Can you work these out from the model? Positions are in its coordinate system, mm. A direction names the side the tool comes from. Round coordinates to 2 decimals unless told otherwise and drop trailing zeros. Loops run counter-clockwise (first coordinate to the right, second up) from the corner with the lowest first, then second, coordinate; pieces in that order, holes last. Notation, with made-up numbers: M 80.5,70 L 122.5,70 A21 ccw 122.5,85 Z; hole C 56.25,70.5 d2. An arc over 180 degrees is marked long. Use a Markdown table: item, result. Add a question column.
```python
from build123d import *

# Parameters (mm, degrees)
F1_DEPTH = 12.7
F2_SCALE = 0.66


with BuildPart() as f1:
    # F0 (on Top) → F1 (new body)
    with BuildSketch(Plane.XY):
        with BuildLine():
            ThreePointArc((9.144, -75.649370546), (57.0228585744, -50.545361805), (76.2, 0))
            ThreePointArc((76.2, 0), (-50.545361805, 57.0228585744), (-9.144, -75.649370546))
            Line((-9.144, -75.649370546), (-9.144, -25.8135372295))
            add(Edge.make_bspline(
                [(-39.7183440202, 0.7753508904), (-39.4440910843, -2.777005422), (-36.553083053, -17.1021078443), (-18.9419593371, -23.7369574995), (-9.144, -25.8135372295)],
                knots=[0, 0, 0, 0, 0.4252369996, 1, 1, 1, 1], degree=3))
            ThreePointArc((-39.7183440202, 0.7753508904), (-40.6754742648, 1.1288974537), (-41.6068021603, 1.5456969604))
            ThreePointArc((-41.6068021603, 1.5456969604), (-48.8665814514, 9.0976146242), (-49.5365875824, 19.5516543956))
            Line((-49.5365875824, 19.5516543956), (-49.7281257293, 19.6451915248))
            Line((-49.7281257293, 19.6451915248), (-48.6135298352, 21.9275753647))
            Line((-48.6135298352, 21.9275753647), (-47.4989339411, 24.2099592047))
            Line((-47.4989339411, 24.2099592047), (-47.3073957942, 24.1164220755))
            ThreePointArc((-47.3073957942, 24.1164220755), (-38.6511413432, 30.0160080471), (-28.2316514308, 28.9343030396))
            ThreePointArc((-28.2316514308, 28.9343030396), (-21.9929696312, 23.3127613442), (-19.6792267956, 15.24))
            ThreePointArc((-19.6792267956, 15.24), (-20.0706784099, 11.8080601931), (-21.2249237559, 8.5524246353))
            ThreePointArc((-21.2249237559, 8.5524246353), (-21.7640042988, 7.5459944723), (-22.3769164732, 6.5827457137))
            add(Edge.make_bspline(
                [(-22.3769164732, 6.5827457137), (-22.3404298332, 0), (-20.8266819608, -2.6844598977), (-13.5609207024, -6.2294838744), (-9.144, -7.5255372295)],
                knots=[0, 0, 0, 0, 0.4802663243, 1, 1, 1, 1], degree=3))
            Line((-9.144, -7.5255372295), (-9.144, 33.528))
            ThreePointArc((-9.144, 33.528), (-9.9126399717, 34.1442853875), (-10.6398545697, 34.8089462134))
            ThreePointArc((-10.6398545697, 34.8089462134), (-15.2387934395, 45.5282331947), (-10.9110537866, 56.3598545697))
            ThreePointArc((-10.9110537866, 56.3598545697), (-1.4654583891, 60.8893780924), (8.6725291214, 58.2517532149))
            Line((8.6725291214, 58.2517532149), (8.8213456053, 58.4043628816))
            Line((8.8213456053, 58.4043628816), (10.6398545697, 56.6310537866))
            Line((10.6398545697, 56.6310537866), (12.4583635342, 54.8577446917))
            Line((12.4583635342, 54.8577446917), (12.3095470503, 54.705135025))
            ThreePointArc((12.3095470503, 54.705135025), (14.4888767171, 50.445468387), (15.24, 45.72))
            ThreePointArc((15.24, 45.72), (14.1163391095, 39.9766063912), (10.9110537866, 35.0801454303))
            ThreePointArc((10.9110537866, 35.0801454303), (10.0575138307, 34.2699338192), (9.144, 33.528))
            Line((9.144, 33.528), (9.144, -40.114004193))
            add(Edge.make_bspline(
                [(24.2416173395, -26.1141094488), (23.9760214951, -29.019635992), (22.6618021702, -35.5712830239), (16.637557432, -36.5809902221), (9.144, -40.114004193)],
                knots=[0, 0, 0, 0, 0.4233523174, 1, 1, 1, 1], degree=3))
            ThreePointArc((24.2416173395, -26.1141094488), (23.4197381725, -25.2409680236), (22.6690500874, -24.305912564))
            ThreePointArc((22.6690500874, -24.305912564), (19.8464755228, -12.9883852305), (25.8533142316, -2.9898232918))
            ThreePointArc((25.8533142316, -2.9898232918), (35.902476764, -0.0317515966), (45.4870784954, -4.2591935428))
            Line((45.4870784954, -4.2591935428), (45.6584180764, -4.132391318))
            Line((45.6584180764, -4.132391318), (47.1694035038, -6.174087436))
            Line((47.1694035038, -6.174087436), (48.6803889311, -8.2157835541))
            Line((48.6803889311, -8.2157835541), (48.50904935, -8.3425857789))
            ThreePointArc((48.50904935, -8.3425857789), (49.7409422113, -11.6939667042), (50.1592267956, -15.24))
            ThreePointArc((50.1592267956, -15.24), (48.5284535825, -22.0990484954), (43.9851393595, -27.4901767082))
            ThreePointArc((43.9851393595, -27.4901767082), (42.9852650291, -28.1704534806), (41.9345988887, -28.76930724))
            add(Edge.make_bspline(
                [(41.9345988887, -28.76930724), (39.9279943087, -35.8152130856), (35.9444698061, -49.8603623611), (18.2756100818, -55.6743562626), (10.5421582828, -58.6083281826), (9.144, -66.9293478131)],
                knots=[0, 0, 0, 0, 0.3663724735, 0.6899474477, 1, 1, 1, 1], degree=3))
            Line((9.144, -66.9293478131), (9.144, -75.649370546))
        make_face()
        with BuildLine():
            ThreePointArc((-42.246771676, 15.991692773), (-41.3581076897, 11.6624633013), (-38.1515548885, 8.6210868642))
            ThreePointArc((-38.1515548885, 8.6210868642), (-32.5245495467, 8.274120524), (-28.3003136597, 12.007671907))
            ThreePointArc((-28.3003136597, 12.007671907), (-27.7424284092, 13.5812290933), (-27.5532267956, 15.24))
            ThreePointArc((-27.5532267956, 15.24), (-28.6715358328, 19.1418346497), (-31.6868987026, 21.8589131358))
            ThreePointArc((-31.6868987026, 21.8589131358), (-36.057035247, 22.5175921793), (-40.0175798878, 20.5564604529))
            ThreePointArc((-40.0175798878, 20.5564604529), (-40.869813648, 19.5814827089), (-41.5381399314, 18.472328093))
            ThreePointArc((-41.5381399314, 18.472328093), (-42.0019035987, 17.2632758839), (-42.246771676, 15.991692773))
        make_face()
        with BuildLine():
            ThreePointArc((-5.2736759969, 50.8625963754), (-7.3654168291, 45.6273127108), (-5.1425963754, 40.4463240031))
            ThreePointArc((-5.1425963754, 40.4463240031), (0.0926872892, 38.3545831709), (5.2736759969, 40.5774036246))
            ThreePointArc((5.2736759969, 40.5774036246), (6.8228972363, 42.9440264224), (7.366, 45.72))
            ThreePointArc((7.366, 45.72), (7.1836656788, 47.3487735922), (6.6456895426, 48.8969114725))
            ThreePointArc((6.6456895426, 48.8969114725), (5.9866540395, 50.0116115169), (5.1425963754, 50.9936759969))
            ThreePointArc((5.1425963754, 50.9936759969), (4.1396028034, 51.8127534522), (3.0086716137, 52.4435296624))
            ThreePointArc((3.0086716137, 52.4435296624), (-1.3810860685, 52.9553684959), (-5.2736759969, 50.8625963754))
        make_face()
        with BuildLine():
            ThreePointArc((28.9983080533, -19.6218577393), (33.8309463237, -22.5251631152), (39.3010845348, -21.1609187423))
            ThreePointArc((39.3010845348, -21.1609187423), (41.4970197426, -18.5552067728), (42.2852267956, -15.24))
            ThreePointArc((42.2852267956, -15.24), (42.2105358085, -14.1936879636), (41.9879775755, -13.1685950634))
            ThreePointArc((41.9879775755, -13.1685950634), (41.5160007505, -11.962725311), (40.8401455379, -10.8581422607))
            ThreePointArc((40.8401455379, -10.8581422607), (39.9812997643, -9.888983904), (38.9660067208, -9.0852028274))
            ThreePointArc((38.9660067208, -9.0852028274), (34.7149131509, -7.8768341093), (30.5373690563, -9.3190812577))
            ThreePointArc((30.5373690563, -9.3190812577), (27.6340636804, -14.1517195281), (28.9983080533, -19.6218577393))
        make_face()
        with BuildLine():
            ThreePointArc((-48.6135298352, 21.9275753647), (-49.1248182042, 20.7589467049), (-49.5365875824, 19.5516543956))
            Line((-49.5365875824, 19.5516543956), (-42.246771676, 15.991692773))
            ThreePointArc((-42.246771676, 15.991692773), (-42.0019035987, 17.2632758839), (-41.5381399314, 18.472328093))
            Line((-41.5381399314, 18.472328093), (-48.6135298352, 21.9275753647))
        make_face()
        with BuildLine():
            ThreePointArc((47.1694035038, -6.174087436), (46.3683450919, -5.1814071443), (45.4870784954, -4.2591935428))
            Line((45.4870784954, -4.2591935428), (38.9660067208, -9.0852028274))
            ThreePointArc((38.9660067208, -9.0852028274), (39.9812997643, -9.888983904), (40.8401455379, -10.8581422607))
            Line((40.8401455379, -10.8581422607), (47.1694035038, -6.174087436))
        make_face()
        with BuildLine():
            Line((41.9879775755, -13.1685950634), (48.50904935, -8.3425857789))
            ThreePointArc((48.50904935, -8.3425857789), (47.8846418194, -7.230280076), (47.1694035038, -6.174087436))
            Line((47.1694035038, -6.174087436), (40.8401455379, -10.8581422607))
            ThreePointArc((40.8401455379, -10.8581422607), (41.5160007505, -11.962725311), (41.9879775755, -13.1685950634))
        make_face()
        with BuildLine():
            Line((6.6456895426, 48.8969114725), (12.3095470503, 54.705135025))
            ThreePointArc((12.3095470503, 54.705135025), (11.5150357988, 55.7030631848), (10.6398545697, 56.6310537866))
            Line((10.6398545697, 56.6310537866), (5.1425963754, 50.9936759969))
            ThreePointArc((5.1425963754, 50.9936759969), (5.9866540395, 50.0116115169), (6.6456895426, 48.8969114725))
        make_face()
        with BuildLine():
            ThreePointArc((10.6398545697, 56.6310537866), (9.6901345511, 57.48260568), (8.6725291214, 58.2517532149))
            Line((8.6725291214, 58.2517532149), (3.0086716137, 52.4435296624))
            ThreePointArc((3.0086716137, 52.4435296624), (4.1396028034, 51.8127534522), (5.1425963754, 50.9936759969))
            Line((5.1425963754, 50.9936759969), (10.6398545697, 56.6310537866))
        make_face()
        with BuildLine():
            ThreePointArc((-47.3073957942, 24.1164220755), (-48.006304368, 23.0493534056), (-48.6135298352, 21.9275753647))
            Line((-48.6135298352, 21.9275753647), (-41.5381399314, 18.472328093))
            ThreePointArc((-41.5381399314, 18.472328093), (-40.869813648, 19.5814827089), (-40.0175798878, 20.5564604529))
            Line((-40.0175798878, 20.5564604529), (-47.3073957942, 24.1164220755))
        make_face()
        with BuildLine():
            ThreePointArc((47.1694035038, -6.174087436), (47.8846418194, -7.230280076), (48.50904935, -8.3425857789))
            Line((48.50904935, -8.3425857789), (48.6803889311, -8.2157835541))
            Line((48.6803889311, -8.2157835541), (47.1694035038, -6.174087436))
        make_face()
        with BuildLine():
            Line((45.6584180764, -4.132391318), (45.4870784954, -4.2591935428))
            ThreePointArc((45.4870784954, -4.2591935428), (46.3683450919, -5.1814071443), (47.1694035038, -6.174087436))
            Line((47.1694035038, -6.174087436), (45.6584180764, -4.132391318))
        make_face()
        with BuildLine():
            Line((8.8213456053, 58.4043628816), (8.6725291214, 58.2517532149))
            ThreePointArc((8.6725291214, 58.2517532149), (9.6901345511, 57.48260568), (10.6398545697, 56.6310537866))
            Line((10.6398545697, 56.6310537866), (8.8213456053, 58.4043628816))
        make_face()
        with BuildLine():
            ThreePointArc((10.6398545697, 56.6310537866), (11.5150357988, 55.7030631848), (12.3095470503, 54.705135025))
            Line((12.3095470503, 54.705135025), (12.4583635342, 54.8577446917))
            Line((12.4583635342, 54.8577446917), (10.6398545697, 56.6310537866))
        make_face()
        with BuildLine():
            Line((-49.7281257293, 19.6451915248), (-49.5365875824, 19.5516543956))
            ThreePointArc((-49.5365875824, 19.5516543956), (-49.1248182042, 20.7589467049), (-48.6135298352, 21.9275753647))
            Line((-48.6135298352, 21.9275753647), (-49.7281257293, 19.6451915248))
        make_face()
        with BuildLine():
            Line((-47.4989339411, 24.2099592047), (-48.6135298352, 21.9275753647))
            ThreePointArc((-48.6135298352, 21.9275753647), (-48.006304368, 23.0493534056), (-47.3073957942, 24.1164220755))
            Line((-47.3073957942, 24.1164220755), (-47.4989339411, 24.2099592047))
        make_face()
    extrude(amount=F1_DEPTH)


with BuildPart() as f1_1:
    # F2: moved
    add(f1.part.scale(F2_SCALE))


solid = f1_1.part
```
(1) Suppose I cut it at A-A on x = 0. List the corners of the cut face in (y, z) for me, and give its area (3 significant figures).
(2) Thinking about a two-plate mould opening in X: for faces 4 (the face through (-30.322, 11.746, 4.132)), 5 (the face through (-6.035, -34, 4)), 6 (the face through (10, 1, 0)), which applies, released by +X, released by -X, zero draft, split by the parting line, or undercut?
(3) On a 3-axis mill with a long thin cutter (end or side, diameter ignored), from which of +Z, -Z, +X, -X, +Y, -Y can I reach the whole of each face in a straight line? I mean faces 1 (the face through (3.881, 36.556, 4.132)), 2 (the face through (-6.035, 8, 4)), 3 (the face through (10, 1, 8.382)). Say none if no direction works.
(4) If I drill on probe 1 along X at (y, z) = (6, 2.5); probe 2 along Y at (x, z) = (15, 1.5); probe 3 along X at (y, z) = (30, 7), over which ranges is the centre line in solid material (lowest first)? Write a range as [from, to].
(5) I'm going to push flat-ended pins straight in: pin 1 (4 mm diameter, centred on x = -1.5, z = 1, fed in from -Y); pin 2 (3 mm diameter, centred on y = -46, z = 3.5, fed in from -X); pin 3 (4 mm diameter, centred on y = -11.5, z = 2.5, fed in from -X); pin 4 (4 mm diameter, centred on x = 34, y = 5.5, fed in from -Z). Where does each tip first touch, or does it pass through?
Results below:
| question | item | result |
|---|---|---|
| 1 | outline | M 25.31,0 L 35.04,0 L 35.04,8.38 L 25.31,8.38 Z; M 40.23,0 L 50.29,0 L 50.29,8.38 L 40.23,8.38 Z |
| 1 | area | 166 mm² |
| 2 | face 4 | undercut |
| 2 | face 5 | undercut |
| 2 | face 6 | zero draft |
| 3 | face 1 | +Z, -Z |
| 3 | face 2 | +Z, -Z, -Y |
| 3 | face 3 | +Z, +X, -X, +Y, -Y |
| 4 | probe 1 | x = [-49.93, -32.25], [-25.72, -20.37], [-13.84, -6.04], [6.04, 49.93] |
| 4 | probe 2 | y = [-48, -35.78], [-21.42, -16.09], [-4.02, 48] |
| 4 | probe 3 | x = [-40.36, -10.06], [-4.86, 4.86], [10.06, 40.36] |
| 5 | pin 1 | stops at y = 25.31 |
| 5 | pin 2 | stops at x = -23.43 |
| 5 | pin 3 | stops at x = -49.39 |
| 5 | pin 4 | stops at z = 0 |
